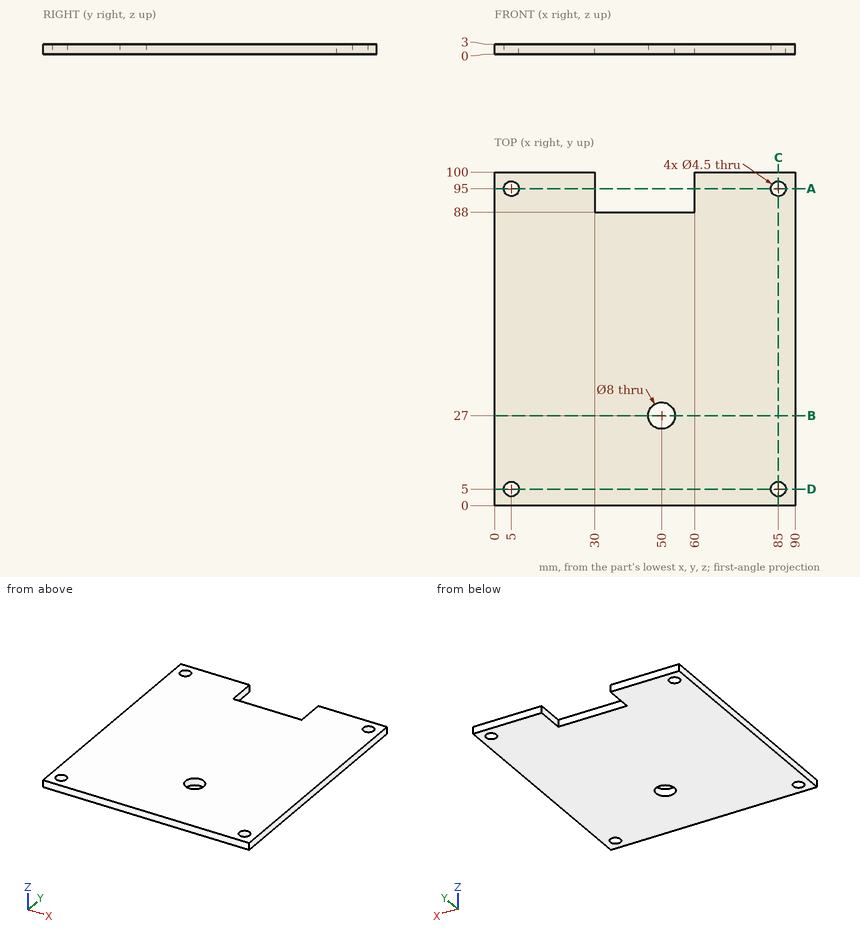
Could you check a few things on this drawing? It's one solid part, dimensions in mm from its lowest x, y, z. Give positions to 0.01 mm unless a question says otherwise; leave off trailing zeros. Order: outer loops, then holes, each group sorted by start corner. A loop starts at its lowest first (then second) coordinate and runs counter-clockwise, first axis right, second up. Notation, with made-up numbers: (56, 43) -> (99, 43) arc R13 ccw to (99, 52) -> close; hole circle Ø1 at (54.25, 70). An arc over 180 degrees is marked (long way). Answer in a Markdown table with one row per item. Add a question column.
Item 1: Imagine slicing it at B-B (y = 27). List the corners of the cut face in (x, z) for me, and give its area (3 significant figures).
Item 2: Please list where these lines run through material, in increasing order: probe 1 along X at (y, z) = (5, 1); probe 2 along Y at (x, z) = (5, 1.85); probe 3 along X at (y, z) = (95, 1.05).
Item 3: Imagine slicing it at D-D (y = 5). List the corners of the cut face in (x, z) for me, and give its area (3 significant figures).
Item 4: Imagine slicing it at C-C (x = 85). List the corners of the cut face in (y, z) for me.
Item 5: I'm going to push flat-ended pins straight in: P1, Ø0.9, axis at y = 94, z = 1, coming from the -X side; P2, Ø0.9, axis at x = 45, z = 1, coming from the +Y side. Where does each tip first touch, or does it pass through?
Item 6: Imagine slicing it at A-A (y = 95). List the corners of the cut face in (x, z) for me.
Result:
| question | item | result |
|---|---|---|
| 1 | outline | (0, 0) -> (46, 0) -> (46, 3) -> (0, 3) -> close; (54, 0) -> (90, 0) -> (90, 3) -> (54, 3) -> close |
| 1 | area | 246 mm2 |
| 2 | probe 1 | 0 to 2.75, 7.25 to 82.75, 87.25 to 90 |
| 2 | probe 2 | 0 to 2.75, 7.25 to 92.75, 97.25 to 100 |
| 2 | probe 3 | 0 to 2.75, 7.25 to 30, 60 to 82.75, 87.25 to 90 |
| 3 | outline | (0, 0) -> (2.75, 0) -> (2.75, 3) -> (0, 3) -> close; (7.25, 0) -> (82.75, 0) -> (82.75, 3) -> (7.25, 3) -> close; (87.25, 0) -> (90, 0) -> (90, 3) -> (87.25, 3) -> close |
| 3 | area | 243 mm2 |
| 4 | outline | (0, 0) -> (2.75, 0) -> (2.75, 3) -> (0, 3) -> close; (7.25, 0) -> (92.75, 0) -> (92.75, 3) -> (7.25, 3) -> close; (97.25, 0) -> (100, 0) -> (100, 3) -> (97.25, 3) -> close |
| 5 | P1 | x = 0 |
| 5 | P2 | y = 88 |
| 6 | outline | (0, 0) -> (2.75, 0) -> (2.75, 3) -> (0, 3) -> close; (7.25, 0) -> (30, 0) -> (30, 3) -> (7.25, 3) -> close; (60, 0) -> (82.75, 0) -> (82.75, 3) -> (60, 3) -> close; (87.25, 0) -> (90, 0) -> (90, 3) -> (87.25, 3) -> close |
